For this review, take the finished solid that the model builds, in its own axes (mm). Face numbers are marked on the shaded views. A direction names the side the tool comes from. Round coordinates to 2 decimals unless told otherwise and drop trailing zeros. Order: outer loops, then holes, each group sorted by start corner. A loop starts at its lowest first (then second) coordinate and runs counter-clockwise, first axis right, second up. Notation, with made-up numbers: M -25.5,-39.5 L 2.5,-39.5 A28 ccw 2.5,-11.5 Z; hole C 3.5,29.25 d9. An arc over 180 degrees is marked long. Use a Markdown table: item, result.
from build123d import *

# Parameters (mm, degrees)
BOSS_EXTRUDE1_DEPTH = 2.5
BOSS_EXTRUDE3_DEPTH = 26.5
BOSS_EXTRUDE5_DEPTH = 29
SKETCH2_R           = 4.5
SKETCH2_R_2         = 1.5
BOSS_EXTRUDE6_DEPTH = 24
FILLET1_R           = 5
CUT_EXTRUDE1_DEPTH  = 10
SKETCH4_R           = 0.7
BOSS_EXTRUDE8_DEPTH = 5
CUT_EXTRUDE3_REACH  = 155
BOSS_EXTRUDE9_DEPTH = 12


with BuildPart() as part:
    # Sketch1 → Boss-Extrude1 (new body)
    with BuildSketch(Plane.XY):
        with BuildLine():
            Line((-70, 72.5), (70, 72.5))
            ThreePointArc((70, 72.5), (82.374368671, 67.374368671), (87.5, 55))
            Line((87.5, 55), (87.5, -55))
            ThreePointArc((87.5, -55), (82.374368671, -67.374368671), (70, -72.5))
            Line((70, -72.5), (-70, -72.5))
            ThreePointArc((-70, -72.5), (-82.374368671, -67.374368671), (-87.5, -55))
            Line((-87.5, -55), (-87.5, 55))
            ThreePointArc((-87.5, 55), (-82.374368671, 67.374368671), (-70, 72.5))
        make_face()
    extrude(amount=BOSS_EXTRUDE1_DEPTH)

    # Sketch1_4 → Boss-Extrude3 (add)
    with BuildSketch(Plane.XY):
        with BuildLine():
            Line((-70, 75), (70, 75))
            ThreePointArc((70, 75), (84.142135624, 69.142135624), (90, 55))
            Line((90, 55), (90, -55))
            ThreePointArc((90, -55), (84.142135624, -69.142135624), (70, -75))
            Line((70, -75), (-70, -75))
            ThreePointArc((-70, -75), (-84.142135624, -69.142135624), (-90, -55))
            Line((-90, -55), (-90, 55))
            ThreePointArc((-90, 55), (-84.142135624, 69.142135624), (-70, 75))
        make_face()
        with BuildLine():
            Line((-70, 72.5), (70, 72.5))
            ThreePointArc((70, 72.5), (82.374368671, 67.374368671), (87.5, 55))
            Line((87.5, 55), (87.5, -55))
            ThreePointArc((87.5, -55), (82.374368671, -67.374368671), (70, -72.5))
            Line((70, -72.5), (-70, -72.5))
            ThreePointArc((-70, -72.5), (-82.374368671, -67.374368671), (-87.5, -55))
            Line((-87.5, -55), (-87.5, 55))
            ThreePointArc((-87.5, 55), (-82.374368671, 67.374368671), (-70, 72.5))
        make_face(mode=Mode.SUBTRACT)
    extrude(amount=BOSS_EXTRUDE3_DEPTH)

    # Sketch1_6 → Boss-Extrude5 (add)
    with BuildSketch(Plane.XY):
        with BuildLine():
            Line((-70, 76.5), (70, 76.5))
            ThreePointArc((70, 76.5), (85.202795796, 70.202795796), (91.5, 55))
            Line((91.5, 55), (91.5, -55))
            ThreePointArc((91.5, -55), (85.202795796, -70.202795796), (70, -76.5))
            Line((70, -76.5), (-70, -76.5))
            ThreePointArc((-70, -76.5), (-85.202795796, -70.202795796), (-91.5, -55))
            Line((-91.5, -55), (-91.5, 55))
            ThreePointArc((-91.5, 55), (-85.202795796, 70.202795796), (-70, 76.5))
        make_face()
        with BuildLine():
            Line((-70, 75), (70, 75))
            ThreePointArc((70, 75), (84.142135624, 69.142135624), (90, 55))
            Line((90, 55), (90, -55))
            ThreePointArc((90, -55), (84.142135624, -69.142135624), (70, -75))
            Line((70, -75), (-70, -75))
            ThreePointArc((-70, -75), (-84.142135624, -69.142135624), (-90, -55))
            Line((-90, -55), (-90, 55))
            ThreePointArc((-90, 55), (-84.142135624, 69.142135624), (-70, 75))
        make_face(mode=Mode.SUBTRACT)
    extrude(amount=BOSS_EXTRUDE5_DEPTH)

    # Sketch2 → Boss-Extrude6 (add)
    with BuildSketch(Plane.XY.offset(2.5)):
        with BuildLine():
            ThreePointArc((82.5, 63), (81.181980515, 59.818019485), (78, 58.5))
            Line((78, 58.5), (87.5, 55))
            ThreePointArc((87.5, 55), (82.374368671, 67.374368671), (70, 72.5))
            Line((70, 72.5), (73.5, 63))
            ThreePointArc((73.5, 63), (78, 67.5), (82.5, 63))
        make_face()
        with Locations((78, 63)):
            Circle(SKETCH2_R)
        with Locations((78, 63)):
            Circle(SKETCH2_R_2, mode=Mode.SUBTRACT)
        with Locations((78, -63)):
            Circle(SKETCH2_R)
        with Locations((78, -63)):
            Circle(SKETCH2_R_2, mode=Mode.SUBTRACT)
        with BuildLine():
            Line((87.5, -55), (78, -58.5))
            ThreePointArc((78, -58.5), (81.181980515, -59.818019485), (82.5, -63))
            ThreePointArc((82.5, -63), (78, -67.5), (73.5, -63))
            Line((73.5, -63), (70, -72.5))
            ThreePointArc((70, -72.5), (82.374368671, -67.374368671), (87.5, -55))
        make_face()
        with Locations((-78, 63)):
            Circle(SKETCH2_R)
        with Locations((-78, 63)):
            Circle(SKETCH2_R_2, mode=Mode.SUBTRACT)
        with BuildLine():
            ThreePointArc((-78, 58.5), (-81.181980515, 66.181980515), (-73.5, 63))
            Line((-73.5, 63), (-70, 72.5))
            ThreePointArc((-70, 72.5), (-82.374368671, 67.374368671), (-87.5, 55))
            Line((-87.5, 55), (-78, 58.5))
        make_face()
        with BuildLine():
            Line((-70, -72.5), (-73.5, -63))
            ThreePointArc((-73.5, -63), (-81.181980515, -66.181980515), (-78, -58.5))
            Line((-78, -58.5), (-87.5, -55))
            ThreePointArc((-87.5, -55), (-82.374368671, -67.374368671), (-70, -72.5))
        make_face()
        with Locations((-78, -63)):
            Circle(SKETCH2_R)
        with Locations((-78, -63)):
            Circle(SKETCH2_R_2, mode=Mode.SUBTRACT)
    extrude(amount=BOSS_EXTRUDE6_DEPTH)

    # Fillet1
    fillet1_edges = [part.edges().sort_by_distance(p)[0] for p in [
        (-85.202795796, 70.202795796, 0),
        (-91.5, 0, 0),
        (-85.202795796, -70.202795796, 0),
        (0, -76.5, 0),
        (85.202795796, -70.202795796, 0),
        (0, 76.5, 0),
        (85.202795796, 70.202795796, 0),
        (91.5, 0, 0),
    ]]
    fillet(fillet1_edges, radius=FILLET1_R)

    # Sketch3 → Cut-Extrude1 (cut)
    with BuildSketch(Plane.XZ.offset(76.5)):
        with BuildLine():
            Line((-5, 12.11379287), (-5, 34.915327667))
            ThreePointArc((-5, 34.915327667), (0, 39.915327667), (5, 34.915327667))
            Line((5, 34.915327667), (5, 12.11379287))
            ThreePointArc((5, 12.11379287), (0, 7.11379287), (-5, 12.11379287))
        make_face()
    extrude(amount=-CUT_EXTRUDE1_DEPTH, mode=Mode.SUBTRACT)

    # Sketch4 → Boss-Extrude8 (add)
    with BuildSketch(Plane.XY.offset(2.5)):
        with BuildLine():
            Line((14.887123517, 10.5), (-14.887123517, 10.5))
            ThreePointArc((-14.887123517, 10.5), (-20.61629509, 9.88370491), (-20, 15.612876483))
            Line((-20, 15.612876483), (-20, 65.387123517))
            ThreePointArc((-20, 65.387123517), (-20.61629509, 71.11629509), (-14.887123517, 70.5))
            Line((-14.887123517, 70.5), (14.887123517, 70.5))
            ThreePointArc((14.887123517, 70.5), (20.61629509, 71.11629509), (20, 65.387123517))
            Line((20, 65.387123517), (20, 15.612876483))
            ThreePointArc((20, 15.612876483), (20.61629509, 9.88370491), (14.887123517, 10.5))
        make_face()
        with Locations((18, 12.5)):
            Circle(SKETCH4_R, mode=Mode.SUBTRACT)
        with Locations((-18, 12.5)):
            Circle(SKETCH4_R, mode=Mode.SUBTRACT)
        with Locations((-18, 68.5)):
            Circle(SKETCH4_R, mode=Mode.SUBTRACT)
        with Locations((18, 68.5)):
            Circle(SKETCH4_R, mode=Mode.SUBTRACT)
        with BuildLine():
            Line((11.42048634, 12.5), (-11.42048634, 12.5))
            ThreePointArc((-11.42048634, 12.5), (-13.381138233, 13.013476781), (-14.838415514, 14.422077922))
            ThreePointArc((-14.838415514, 14.422077922), (-15.38370491, 15.11629509), (-16.077922078, 15.661584486))
            ThreePointArc((-16.077922078, 15.661584486), (-17.486523219, 17.118861767), (-18, 19.07951366))
            Line((-18, 19.07951366), (-18, 61.92048634))
            ThreePointArc((-18, 61.92048634), (-17.486523219, 63.881138233), (-16.077922078, 65.338415514))
            ThreePointArc((-16.077922078, 65.338415514), (-15.38370491, 65.88370491), (-14.838415514, 66.577922078))
            ThreePointArc((-14.838415514, 66.577922078), (-13.381138233, 67.986523219), (-11.42048634, 68.5))
            Line((-11.42048634, 68.5), (11.42048634, 68.5))
            ThreePointArc((11.42048634, 68.5), (13.381138233, 67.986523219), (14.838415514, 66.577922078))
            ThreePointArc((14.838415514, 66.577922078), (15.38370491, 65.88370491), (16.077922078, 65.338415514))
            ThreePointArc((16.077922078, 65.338415514), (17.486523219, 63.881138233), (18, 61.92048634))
            Line((18, 61.92048634), (18, 19.07951366))
            ThreePointArc((18, 19.07951366), (17.486523219, 17.118861767), (16.077922078, 15.661584486))
            ThreePointArc((16.077922078, 15.661584486), (15.38370491, 15.11629509), (14.838415514, 14.422077922))
            ThreePointArc((14.838415514, 14.422077922), (13.381138233, 13.013476781), (11.42048634, 12.5))
        make_face(mode=Mode.SUBTRACT)
    extrude(amount=BOSS_EXTRUDE8_DEPTH)

    # Sketch5 → Cut-Extrude3 (cut, up to next)
    with BuildSketch(Plane(origin=(0, 76.5, 0), x_dir=(1, 0, 0), z_dir=(0, 1, 0)), mode=Mode.PRIVATE) as cut_extrude3_sk1:
        with BuildLine():
            Line((10, -25), (-10, -25))
            ThreePointArc((-10, -25), (-17.5, -17.5), (-10, -10))
            Line((-10, -10), (10, -10))
            ThreePointArc((10, -10), (17.5, -17.5), (10, -25))
        make_face()
    cut_extrude3_tool1 = extrude(cut_extrude3_sk1.sketch, amount=-CUT_EXTRUDE3_REACH, mode=Mode.PRIVATE) & part.part
    add(cut_extrude3_tool1.solids().sort_by_distance((0, 76.5, 17.5))[0], mode=Mode.SUBTRACT)

    # Sketch6 → Boss-Extrude9 (add)
    with BuildSketch(Plane.XY.offset(2.5)):
        with BuildLine():
            Line((-21.678083714, 57.14631801), (-25.178083714, 57.14631801))
            Line((-25.178083714, 57.14631801), (-25.178083714, 56.19631801))
            ThreePointArc((-25.178083714, 56.19631801), (-24.378083714, 55.39631801), (-25.178083714, 54.59631801))
            Line((-25.178083714, 54.59631801), (-25.178083714, 53.64631801))
            Line((-25.178083714, 53.64631801), (-25.178083714, 18.64631801))
            Line((-25.178083714, 18.64631801), (-80.178083714, 18.64631801))
            Line((-80.178083714, 18.64631801), (-80.178083714, 17.69631801))
            Line((-80.178083714, 17.69631801), (-25.178083714, 17.69631801))
            ThreePointArc((-25.178083714, 17.69631801), (-24.378083714, 16.89631801), (-25.178083714, 16.09631801))
            Line((-25.178083714, 16.09631801), (-80.178083714, 16.09631801))
            Line((-80.178083714, 16.09631801), (-80.178083714, 15.14631801))
            Line((-80.178083714, 15.14631801), (-21.678083714, 15.14631801))
            Line((-21.678083714, 15.14631801), (-21.678083714, 57.14631801))
        make_face()
        with BuildLine():
            Line((-25.178083714, 56.19631801), (-25.178083714, 57.14631801))
            Line((-25.178083714, 57.14631801), (-81.674279688, 57.14631801))
            Line((-81.674279688, 57.14631801), (-83.678083714, 56.408074421))
            Line((-83.678083714, 56.408074421), (-83.678083714, 15.14631801))
            Line((-83.678083714, 15.14631801), (-80.178083714, 15.14631801))
            Line((-80.178083714, 15.14631801), (-80.178083714, 16.09631801))
            ThreePointArc((-80.178083714, 16.09631801), (-80.978083714, 16.89631801), (-80.178083714, 17.69631801))
            Line((-80.178083714, 17.69631801), (-80.178083714, 18.64631801))
            Line((-80.178083714, 18.64631801), (-80.178083714, 53.64631801))
            Line((-80.178083714, 53.64631801), (-25.178083714, 53.64631801))
            Line((-25.178083714, 53.64631801), (-25.178083714, 54.59631801))
            Line((-25.178083714, 54.59631801), (-80.178083714, 54.59631801))
            ThreePointArc((-80.178083714, 54.59631801), (-80.978083714, 55.39631801), (-80.178083714, 56.19631801))
            Line((-80.178083714, 56.19631801), (-25.178083714, 56.19631801))
        make_face()
    extrude(amount=BOSS_EXTRUDE9_DEPTH)


solid = part.part
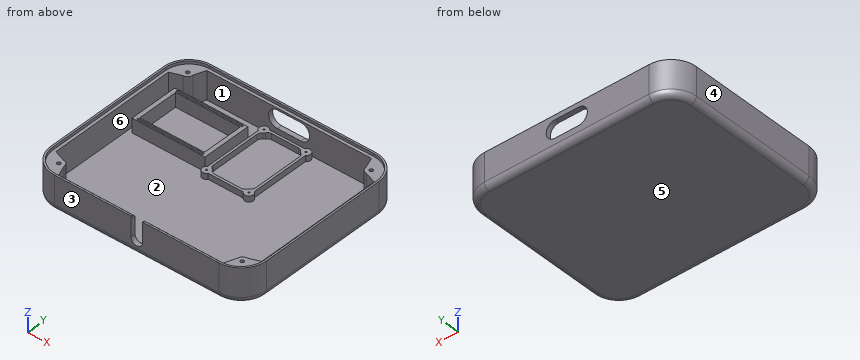
Q1. Add section C-C (z = 17.5). Give the number of separate pieces and of enclosed holes in the cut face, then the cut area to 3 significant figures.
Determined:
| item | result |
|---|---|
| separate pieces | 2 |
| enclosed holes | 4 |
| area | 2,920 mm^2 |
Q2. Draft analysis for pull direction X (two halves, no side actions). For the marked faces 1, 2, 3 and 4, state which applies: pulls with the +X half, pulls with the -X half, needs draft (parallel to the pull), parting line crosses it, or undercut.
Determined:
| item | result |
|---|---|
| face 1 | undercut |
| face 2 | undercut |
| face 3 | needs draft |
| face 4 | pulls with the -X half |
Q3. Wall thickness on line 1 along Y through (x, z) = (-48.5, 14.25); line 2 along X through (y, z) = (2, 23.75); line 3 along X through (y, z) = (-51.5, 27): over which ranges is each line inside the solid? List them lowest first. Write a range as [from, to].
Determined:
| item | result |
|---|---|
| line 1 | y = [-76.5, -72.5], [15.15, 16.1], [17.7, 18.65], [53.65, 54.6], [56.2, 57.15], [72.5, 76.5] |
| line 2 | x = [-91.5, -87.5], [87.5, 91.5] |
| line 3 | x = [-91.5, -90], [90, 91.5] |
Q4. Machinability: for the marked faces 5 and 6, which of the approach directions +Z, -Z, +X, -X, +Y, -Y give a long, thin tool a straight path to every point of the face, cutting with its end or side? Answer none if there is none.
Determined:
| item | result |
|---|---|
| face 5 | -Z, +X, -X, +Y, -Y |
| face 6 | +Z |
Q5. Add section D-D (x = 28.5). Write out the cut boundary in (y, z), then the cut area to 3 significant figures.
Determined:
| item | result |
|---|---|
| outline | M -76.5,5 A5 ccw -71.5,0 L 71.5,0 A5 ccw 76.5,5 L 76.5,29 L 75,29 L 75,26.5 L 72.5,26.5 L 72.5,2.5 L -72.5,2.5 L -72.5,26.5 L -75,26.5 L -75,29 L -76.5,29 Z |
| area | 571 mm^2 |
Q6. Clearance check with flat-ended pins moving along their axes: pin 1 (1.3 mm diameter, centred on x = -18, y = 12.5, fed in from +Z); pin 2 (2 mm diameter, centred on y = -73.5, z = 23, fed in from +X). State where each tip first meets the part, or that it passes through.
Determined:
| item | result |
|---|---|
| pin 1 | stops at z = 2.5 |
| pin 2 | stops at x = 82.49 |
